Verification items for this drawing (mm, ordinates from the low corner). A direction names the side the tool comes from. Round coordinates to 2 decimals unless told otherwise and drop trailing zeros. Loops run counter-clockwise (first coordinate to the right, second up) from the corner with the lowest first, then second, coordinate; pieces in that order, holes last. Notation, with made-up numbers: M 48,7 L 90,7 A26 cw 90,23 Z; hole C 79.25,38 d7. An arc over 180 degrees is marked long. Write item = value, one per line. Start each with the question number.
(1) Go/stop test with a flat-tipped pin: P1, Ø10, axis at x = 14, y = 2, coming from the -Z side (1 decimal). Record where the tip stops, or that it passes through.
(2) Set-up check for the marked faces 1 and 2: record each of +Z, -Z, +X, -X, +Y, -Y from which the full face is reachable in a straight line by a thin tool's end or side.
(3) Cross-section at C-C on z = 10.5. Record the boundary of the cut face in (x, y), plus the area to 3 significant figures.
(4) Scan lines: L1, parallel to Z at x = 23, y = 2.5; L2, parallel to Y at x = 23, z = 18; L3, parallel to X at y = 18.25, z = 11 (1 decimal). Record each from-to range of solid material in increasing order. Write a range as from..to.
(5) Cross-section at B-B on x = 20. Record the boundary of the cut face in (y, z).
(6) Mould release check, pull along X, two halves, no side actions. Record for the marked faces 3, 4 and 5: pulls with the +X half, pulls with the -X half, needs draft (parallel to the pull), parting line crosses it, or undercut.
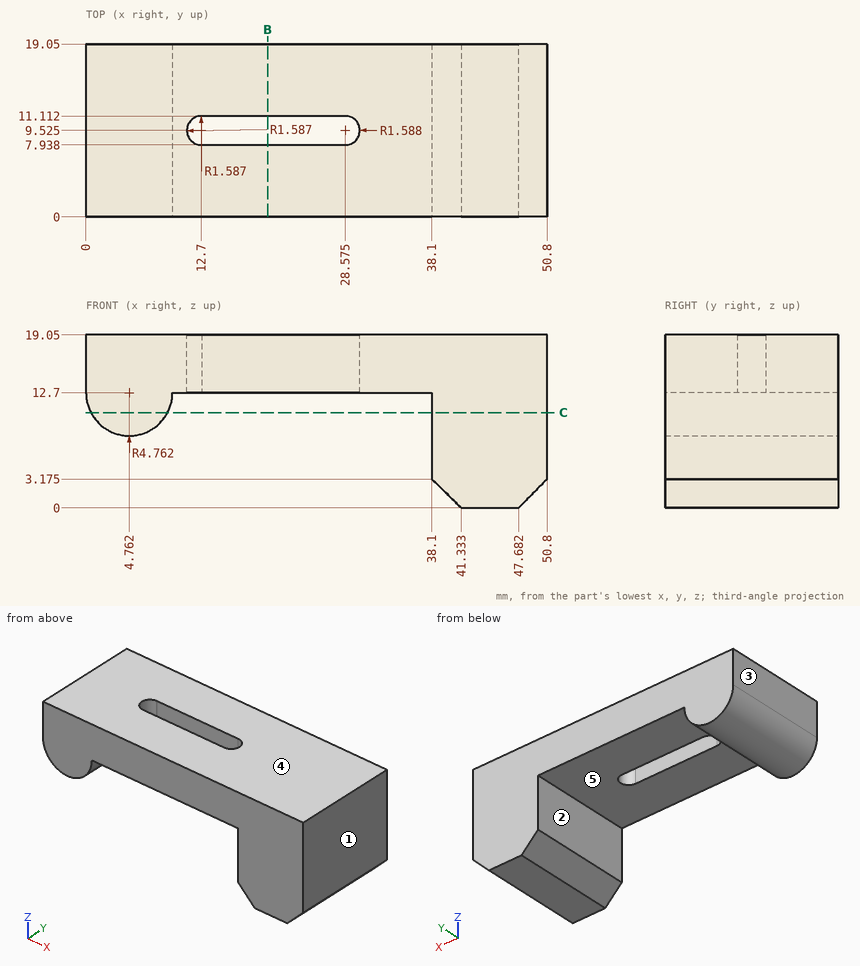
Result:
q1.P1 = 10.5
q2.face_1 = +Z, -Z, +X, +Y, -Y
q2.face_2 = -Z, +Y, -Y
q3.outline = M 0.54,0 L 8.99,0 L 8.99,19.05 L 0.54,19.05 Z; M 38.1,0 L 50.8,0 L 50.8,19.05 L 38.1,19.05 Z
q3.area = 403 mm^2
q4.L1 = 12.7..19.05
q4.L2 = 0..7.94, 11.11..19.05
q4.L3 = 0.3..9.2, 38.1..50.8
q5.outline = M 0,12.7 L 7.94,12.7 L 7.94,19.05 L 0,19.05 Z; M 11.11,12.7 L 19.05,12.7 L 19.05,19.05 L 11.11,19.05 Z
q6.face_3 = pulls with the -X half
q6.face_4 = needs draft
q6.face_5 = undercut
